Could you check a few things on this model? Use its own coordinates, in mm. A direction names the side the tool comes from. Coordinates: 2 decimals unless noted, no trailing zeros. Loops run counter-clockwise (first coordinate to the right, second up) from the corner with the lowest first, then second, coordinate; pieces in that order, holes last. Notation, with made-up numbers: (-29, -13) -> (8, -13) arc R22 ccw to (8, 18) -> close; hole circle Ø8 at (31, 22.5). An arc over 180 degrees is marked (long way). One line per question, with ' | ' between items.
```python
from build123d import *
from build123d.topology import SkipClean

# Parameters (mm, degrees)
BOSS_EXTRUDE1_DEPTH     = 2
MIRROR1_OUTLINE_R       = 1.25
MIRROR1_DEPTH           = 2
SKETCH2_W               = 25
SKETCH2_H               = 1.9
BOSS_EXTRUDE2_DEPTH     = 22
BOSS_EXTRUDE3_REACH     = 34.879
SKETCH3_W               = 25
SKETCH3_H               = 2
CUT_EXTRUDE1_DEPTH      = 31.761176831
CUT_EXTRUDE1_DEPTH_BACK = 3
SKETCH4_R               = 2.5


# Read off the part's stored shape, not the designer's step: Mirror1
with BuildPart() as part:
    # Sketch1 → Boss-Extrude1 (new body)
    with BuildSketch(Plane.XY):
        with BuildLine():
            Line((-17.5, 8), (0, 8))
            Line((0, 8), (0, 6.1))
            Line((0, 6.1), (-12.5, 6.1))
            Line((-12.5, 6.1), (-12.5, 0))
            Line((-12.5, 0), (-13.25, 0))
            ThreePointArc((-13.25, 0), (-14.5, 1.25), (-15.75, 0))
            Line((-15.75, 0), (-17.5, 0))
            Line((-17.5, 0), (-17.5, 8))
        make_face()
    extrude(amount=BOSS_EXTRUDE1_DEPTH)

    # Mirror1 outline → Mirror1 (add)
    with SkipClean():  # the faces are left unmerged after this step: merging them gives an invalid solid
        with BuildSketch(Plane.XY):
            with BuildLine():
                Line((17.5, 8), (0, 8))
                Line((0, 8), (0, 6.1))
                Line((0, 6.1), (12.5, 6.1))
                Line((12.5, 6.1), (12.5, -6.1))
                Line((12.5, -6.1), (-12.5, -6.1))
                Line((-12.5, -6.1), (-12.5, 0))
                Line((-12.5, 0), (-13.25, 0))
                ThreePointArc((-13.25, 0), (-14.5, -1.25), (-15.75, 0))
                Line((-15.75, 0), (-17.5, 0))
                Line((-17.5, 0), (-17.5, -8))
                Line((-17.5, -8), (17.5, -8))
                Line((17.5, -8), (17.5, 8))
            make_face()
            with Locations((14.5, 0)):
                Circle(MIRROR1_OUTLINE_R, mode=Mode.SUBTRACT)
        extrude(amount=MIRROR1_DEPTH)
    add(part.part.scale(1), mode=Mode.REPLACE)  # the faces are merged on a copy

    # Sketch2 → Boss-Extrude2 (add)
    with BuildSketch(Plane.XY.offset(2)):
        with Locations((0, 7.05)):
            Rectangle(SKETCH2_W, SKETCH2_H)
        with Locations((0, -7.05)):
            Rectangle(SKETCH2_W, SKETCH2_H)
    extrude(amount=BOSS_EXTRUDE2_DEPTH)

    # Sketch3 → Boss-Extrude3 (add, up to next)
    with BuildSketch(Plane(origin=(0, -6.1, 0), x_dir=(1, 0, 0), z_dir=(0, 1, 0)), mode=Mode.PRIVATE) as boss_extrude3_sk1:
        with Locations((0, -23)):
            Rectangle(SKETCH3_W, SKETCH3_H)
    boss_extrude3_tool1 = extrude(boss_extrude3_sk1.sketch, amount=BOSS_EXTRUDE3_REACH, mode=Mode.PRIVATE) - part.part
    add(boss_extrude3_tool1.solids().sort_by_distance((0, -6.1, 23))[0])

    # Sketch4 → Cut-Extrude1 (cut, two sides: drawn at the far end of the back side and taken through both)
    with BuildSketch(Plane.XY.offset(24).offset(-CUT_EXTRUDE1_DEPTH_BACK)):
        with Locations(Location((-6.892107872, 0, 0), (0, 0, 180))):
            Circle(SKETCH4_R)
    extrude(amount=CUT_EXTRUDE1_DEPTH + CUT_EXTRUDE1_DEPTH_BACK, mode=Mode.SUBTRACT)


solid = part.part
```
Q1. Imagine slicing it at A-A on x = 14.5. Write out the boundary of the cut face in (y, z), plus the area to 3 significant figures.
Values follow:
outline: (-8, 0) -> (-1.25, 0) -> (-1.25, 2) -> (-8, 2) -> close; (1.25, 0) -> (8, 0) -> (8, 2) -> (1.25, 2) -> close | area: 27.0 mm2
Q2. Please list where these lines run through material, in increasing order: L1, parallel to Y at x = 9, z = 9.75; L2, parallel to Z at x = -13.5, y = -6.5; L3, parallel to Z at x = -1, y = 0.5. Write a range as [from, to].
Values follow:
L1: y = [-8, -6.1], [6.1, 8] | L2: z = [0, 2] | L3: z = [22, 24]
Q3. For pin 1 (4 mm diameter, centred on y = 5, z = 11, fed in from -X); pin 2 (4 mm diameter, centred on x = 2, y = -3, fed in from -Z); pin 3 (1.5 mm diameter, centred on x = 14, y = 2.5, fed in from +Z), each with a flat end and sliding along its axis, tell me the tip position at first contact or that it passes through.
Values follow:
pin 1: stops at x = -12.5 | pin 2: stops at z = 22 | pin 3: stops at z = 2
Q4. Imagine slicing it at B-B on y = -5.5. Write out the boundary of the cut face in (x, z), plus the area to 3 significant figures.
Values follow:
outline: (-17.5, 0) -> (-12.5, 0) -> (-12.5, 2) -> (-17.5, 2) -> close; (-12.5, 22) -> (12.5, 22) -> (12.5, 24) -> (-12.5, 24) -> close; (12.5, 0) -> (17.5, 0) -> (17.5, 2) -> (12.5, 2) -> close | area: 70.0 mm2
Q5. Imagine slicing it at D-D on x = 5. Write out the boundary of the cut face in (y, z).
Values follow:
outline: (-8, 0) -> (-6.1, 0) -> (-6.1, 22) -> (6.1, 22) -> (6.1, 0) -> (8, 0) -> (8, 24) -> (-8, 24) -> close
Q6. For faces 1 (the face through (0, 8, 12)), 2 (the face through (0, 0, 24)), 3 (the face through (-12.5, 0, 1)), 4 (the face through (-16, 0, 2)), 5 (the face through (12.5, -7, 16)), which set-ups out of +Z, -Z, +X, -X, +Y, -Y let a thin tool reach every point of the face, with its end or its side?
Values follow:
face 1: +Z, -Z, +X, -X, +Y | face 2: +Z, +X, -X, +Y, -Y | face 3: -Z | face 4: +Z, -X, +Y, -Y | face 5: +Z, +X, +Y, -Y
Q7. Imagine slicing it at C-C on z = 11.5. Write out the boundary of the cut face in (x, y), plus the area to 3 significant figures.
Values follow:
outline: (-12.5, -8) -> (12.5, -8) -> (12.5, -6.1) -> (-12.5, -6.1) -> close; (-12.5, 6.1) -> (12.5, 6.1) -> (12.5, 8) -> (-12.5, 8) -> close | area: 95.0 mm2
Q8. We'd pull the mould along Y, two halves only. Please class faces 6 (the face through (-12.5, -7, 16)), 7 (the face through (0, -8, 12)), 8 (the face through (-9.277, -0.751, 22.986)), 9 (the face through (0, 0, 22)): released by +Y, released by -Y, zero draft, split by the parting line, or undercut.
Values follow:
face 6: zero draft | face 7: released by -Y | face 8: undercut | face 9: undercut
